```python
from build123d import *

# Parameters (mm, degrees)
SKETCH_1_W          = 10
SKETCH_1_H          = 10
EXTRUDE_1_DEPTH     = 11
SKETCH_2_R          = 5
SKETCH_2_R_2        = 4
EXTRUDE_2_DEPTH     = 20
SKETCH_3_W          = 6
SKETCH_3_H          = 10
CUT_EXTRUDE_1_DEPTH = 60
CUT_EXTRUDE_2_DEPTH = 60


with BuildPart() as part:
    # 草图1 → 凸台-拉伸1 (new body)
    with BuildSketch(Plane(origin=(0, 0, 0), x_dir=(1, 0, 0), z_dir=(0, 1, 0))):
        Rectangle(SKETCH_1_W, SKETCH_1_H)
    extrude(amount=EXTRUDE_1_DEPTH)

    # 草图2 → 凸台-拉伸2 (add)
    with BuildSketch(Plane(origin=(0, 11, 0), x_dir=(1, 0, 0), z_dir=(0, 1, 0))):
        Circle(SKETCH_2_R)
        Circle(SKETCH_2_R_2, mode=Mode.SUBTRACT)
    extrude(amount=EXTRUDE_2_DEPTH)

    # 草图3 → 切除-拉伸1 (cut)
    with BuildSketch(Plane(origin=(5, 0, 0), x_dir=(0, 0, -1), z_dir=(1, 0, 0))):
        with Locations((0, 5)):
            Rectangle(SKETCH_3_W, SKETCH_3_H)
    extrude(amount=-CUT_EXTRUDE_1_DEPTH, mode=Mode.SUBTRACT)

    # 草图4 → 切除-拉伸2 (cut)
    with BuildSketch(Plane.XY.offset(5)):
        with BuildLine():
            Line((-5, 5), (-5, -1.760834605))
            Line((-5, -1.760834605), (5, -1.760834605))
            Line((5, -1.760834605), (5, 5))
            ThreePointArc((5, 5), (0, 0), (-5, 5))
        make_face()
    extrude(amount=-CUT_EXTRUDE_2_DEPTH, mode=Mode.SUBTRACT)


solid = part.part
```
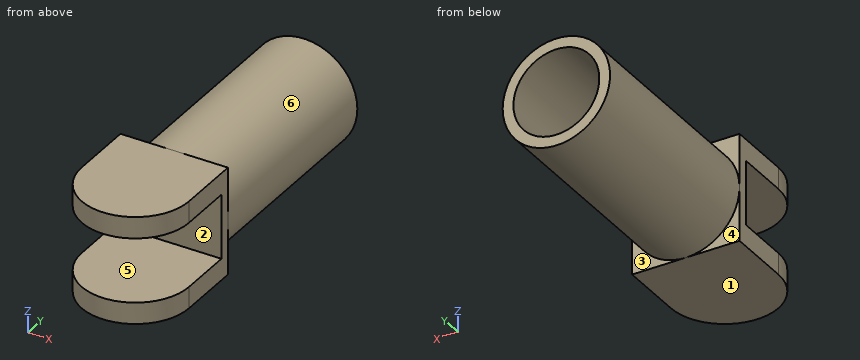
Here's how the part is built. I have some questions about the finished solid (model axes, mm). Face numbers are marked on the shaded views. A direction names the side the tool comes from. Round coordinates to 2 decimals unless told otherwise and drop trailing zeros. Order: outer loops, then holes, each group sorted by start corner. A loop starts at its lowest first (then second) coordinate and runs counter-clockwise, first axis right, second up. Notation, with made-up numbers: (-19.75, 85) -> (0.25, 85) arc R29 cw to (0.25, 106) -> close; hole circle Ø10 at (-38, 25.25). An arc over 180 degrees is marked (long way). Use a Markdown table: item, result. Add a question column.
(1) Suppose I cut it at C-C, the plane y = 24. Please give me the cut outline in (x, z), and give its area (3 significant figures).
(2) Suppose I cut it at A-A, the plane y = 3.5. Please give me the cut outline in (x, z).
(3) I need wall thicknesses on line 1 along Z through (x, y) = (-3.25, 2.5); line 2 along X through (y, z) = (21.25, 0). Which ranges of each line are inside material? Lowest first, please.
(4) For pin 1 Ø2.5 at (x, z) = (1.5, 1) entering from +Y; pin 2 Ø3 at (x, z) = (1.5, 0.5) entering from -Y; pin 3 Ø3 at (y, z) = (16.5, 3.5) entering from +X, each with a flat end and sliding along its axis, tell me the tip position at first contact or that it passes through.
(5) If we mould it in two halves opening along Z, with no side actions, what happens to the marked faces 1, 2 and 3? For each: released by +Z, released by -Z, zero draft, split by the parting line, or undercut.
(6) For the marked faces 4, 5 and 6, which set-ups out of +Z, -Z, +X, -X, +Y, -Y let a thin tool reach every point of the face, with its end or its side?
(7) Suppose I cut it at D-D, the plane x = 2.25. Please give me the cut outline in (y, z).
Verdict:
| question | item | result |
|---|---|---|
| 1 | outline | circle Ø10 at (0, 0); hole circle Ø8 at (0, 0) |
| 1 | area | 28.3 mm2 |
| 2 | outline | (-4.77, -5) -> (4.77, -5) -> (4.77, -3) -> (-4.77, -3) -> close; (-4.77, 3) -> (4.77, 3) -> (4.77, 5) -> (-4.77, 5) -> close |
| 3 | line 1 | -5 to -3, 3 to 5 |
| 3 | line 2 | -5 to -4, 4 to 5 |
| 4 | pin 1 | y = 11 |
| 4 | pin 2 | y = 10 |
| 4 | pin 3 | x = 4.58 |
| 5 | face 1 | released by -Z |
| 5 | face 2 | undercut |
| 5 | face 3 | zero draft |
| 6 | face 4 | -Z, -X, +Y |
| 6 | face 5 | +X, -X, -Y |
| 6 | face 6 | +Y |
| 7 | outline | (0.53, -5) -> (11, -5) -> (11, -4.47) -> (31, -4.47) -> (31, -3.31) -> (11, -3.31) -> (11, 3.31) -> (31, 3.31) -> (31, 4.47) -> (11, 4.47) -> (11, 5) -> (0.53, 5) -> (0.53, 3) -> (10, 3) -> (10, -3) -> (0.53, -3) -> close |
